Source: CAD feature listing. Evaluate the final solid. Frame: model axes, mm. Face numbers are marked on the shaded views. A direction names the side the tool comes from. Coordinates: 2 decimals unless noted, no trailing zeros. Loops run counter-clockwise (first coordinate to the right, second up) from the corner with the lowest first, then second, coordinate; pieces in that order, holes last.
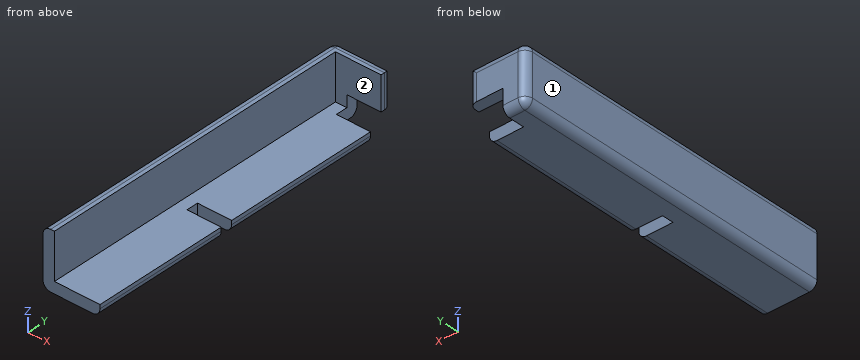
Autodesk Inventor part; units mm, degrees
ref_plane "YZ Plane" through (0, 0, 0) normal (1, 0, 0) x (0, 1, 0)
ref_plane "XZ Plane" through (0, 0, 0) normal (0, 1, 0) x (-1, 0, 0)
ref_plane "XY Plane" through (0, 0, 0) normal (0, 0, 1) x (1, 0, 0)
sketch "Sketch1" plane through (0, 0, 0) normal (0, 1, 0) x (-1, 0, 0)
  line L0 (15, 0) -> (15, -15)
  line L1 (15, -15) -> (0, -15)
  line L2 (0, -15) -> (0, -12)
  line L3 (0, -12) -> (12, -12)
  line L4 (12, -12) -> (12, 0)
  line L5 (12, 0) -> (15, 0)
  point P0 (0, 0)
  dimension "d0" = 15
  dimension "d1" = 15
  dimension "d10" = 3
  dimension "d11" = 12
  dimension "d12" = 12
extrude "Extrusion1" add sketch "Sketch1" along normal blind 86
sketch "Sketch4" plane through (-12, 0, 0) normal (1, 0, 0) x (0, 0, -1)
  line L0 (0, 0) -> (0, 86)
  line L1 (12, 0) -> (12, 86)
  line L2 (0, 86) -> (12, 86)
  line L3 (12, 86) -> (12, 83)
  line L4 (12, 83) -> (0, 83)
  line L5 (0, 83) -> (0, 86)
  dimension "d13" = 3
extrude "Extrusion3" add sketch "Sketch4" along normal blind 3
sketch "Sketch6" plane through (-12, 0, -12) normal (0, 0, 1) x (1, 0, 0)
  line L0 (3, 86) -> (12, 86)
  line L1 (12, 86) -> (3, 86)
  line L2 (3, 86) -> (3, 83)
  line L3 (3, 83) -> (12, 83)
  line L4 (12, 83) -> (12, 86)
  point P0 (12, 0)
extrude "Extrusion4" add sketch "Sketch6" along normal blind 12
fillet "Fillet3" radius 2 7 edges at (-7.5, 86, -15) (-15, 86, -7.5) (-15, 43, -15) (0, 43, -15) (-7.5, 86, 0) (0, 86, -7.5) (-15, 43, 0)
sketch "Sketch11" plane through (0, 86, 0) normal (0, 1, 0) x (1, 0, 0)
  arc A0 (-15, 2) -> (-13, 0) centre (-13, 2) ccw
  line L0 (0, 10.8348) -> (0, 14)
  line L1 (0, 9) -> (0, 10.8348)
  line L2 (-9, 15) -> (0, 15)
  line L3 (0, 15) -> (0, 9)
  line L4 (-9, 15) -> (-9, 9)
  line L5 (-9, 9) -> (-9, 8.9)
  line L6 (-9, 8.9) -> (0, 8.9)
  line L7 (0, 8.9) -> (0, 9)
  point P0 (-13, 0)
  point P1 (0, 15)
extrude "Extrusion7" cut sketch "Sketch11" against normal blind 6.1
sketch "Sketch12" plane through (-12, 0, -12) normal (0, 0, 1) x (1, 0, 0)
  line L0 (12, 33) -> (21, 33) construction
  line L1 (3, 38.9) -> (3, 35.8)
  line L2 (3, 35.8) -> (12, 35.8)
  line L3 (3, 35.8) -> (12, 35.8) construction
  line L4 (12, 35.8) -> (12, 38.9)
  line L5 (12, 79.9) -> (12, 0)
  line L6 (12, 38.9) -> (3, 38.9)
  dimension "d49" = 3.1
extrude "Extrusion8" cut sketch "Sketch12" against normal through all
properties part number "DoosjeHoeken" material "ABS Plastic"
Q1. Section D-D, the plane x = -11. Return the cut outline in (y, z).
Q2. Line query: line 1 along Z through (x, y) = (-8.25, 59); line 2 along Y through (x, z) = (-9.25, -2.5). Output: solid intervals per line, ascending.
Q3. Access query for the marked faces 1 and 2. Directions: +Z, -Z, +X, -X, +Y, -Y. A direction counts if a zero-diameter tool reaches every point of the face in a straight line with its end or side. Return the directions, or none.
Q4. Contact query for flat-ended pins moving along their axis: pin 1 Ø3.5 at (x, z) = (-4, -6.5) entering from -Y; pin 2 Ø2.5 at (x, z) = (-5, -13) entering from +Y; pin 3 Ø6.5 at (y, z) = (83.5, -13) entering from +X. Output: stop coordinate, or through.
Q5. Section C-C, the plane y = 47. Return the cut outline in (x, z), plus the area to 3 significant figures.
Q6. Section B-B, the plane z = -11. Return the cut outline in (x, y), plus the area to 3 significant figures.
Q7. Section A-A, the plane x = -7.75. Return the cut outline in (y, z).
Derived:
1. outline: (0, -15) - (84, -15) arc R2 ccw to (86, -13) - (86, -2) arc R2 ccw to (84, 0) - (83, 0) - (83, -12) - (0, -12) - close
2. line 1: z = -15 to -12
2. line 2: y = 83 to 86
3. face 1: +Z, -Z, -X, +Y, -Y
3. face 2: +Z, +X, -Y
4. pin 1: stops at y = 83
4. pin 2: stops at y = 79.9
4. pin 3: stops at x = -9
5. outline: (-15, -13) arc R2 ccw to (-13, -15) - (-2, -15) arc R2 ccw to (0, -13) - (0, -12) - (-12, -12) - (-12, 0) - (-13, 0) arc R2 ccw to (-15, -2) - close
5. area: 78.4 mm2
6. outline: (-15, 0) - (-12, 0) - (-12, 83) - (-9, 83) - (-9, 86) - (-13, 86) arc R2 ccw to (-15, 84) - close
6. area: 266 mm2
7. outline: (0, -15) - (35.8, -15) - (35.8, -12) - (0, -12) - close; (38.9, -15) - (79.9, -15) - (79.9, -12) - (38.9, -12) - close; (83, -8.9) - (86, -8.9) - (86, -2) arc R2 ccw to (84, 0) - (83, 0) - close
